Geometry: final body of the model. Coordinates: model frame, mm. A direction names the side the tool comes from. Coordinates: 2 decimals unless noted, no trailing zeros. Order: outer loops, then holes, each group sorted by start corner. A loop starts at its lowest first (then second) coordinate and runs counter-clockwise, first axis right, second up. Notation, with made-up numbers: M 72,59.25 L 115,59.25 A7 cw 115,64.25 Z; hole C 3.25,-8 d4. An arc over 180 degrees is marked long. Use CSV: the item, a comma, the result in double quotes. Start each with the question number.
Q1. Access query for faces 1 (the face through (-4, 3, 5.8)), 2 (the face through (0, 0, 0)). Directions: +Z, -Z, +X, -X, +Y, -Y. A direction counts if a zero-diameter tool reaches every point of the face in a straight line with its end or side. Return the directions, or none.
Q2. Section query B-B, the plane z = 2.75. Output: boundary loops of the cut face in (x, y), and give its area (3 significant figures).
Q3. First-contact query: P1, Ø2, axis at x = -4, y = 1.5, coming from the -Z side; P2, Ø3, axis at x = -2.5, y = 3, coming from the +Z side; P3, Ø2, axis at x = -2.5, y = -0.5, coming from the +Z side; P4, Ø6, axis at x = 2, y = 2.5, coming from the -Z side. Flat tips, straight axial feed; report the tip coordinate or a pass-through.
Q4. Section query A-A, the plane x = 0. Output: boundary loops of the cut face in (y, z) (3 decimals).
Q5. Ray query, probe 1 along Z at (x, y) = (3, -4); probe 2 along X at (y, z) = (3.75, 2.25); probe 3 along Y at (x, z) = (1.75, 4.5). Return the intervals inside material, ascending.
Q6. Section query C-C, the plane z = 1. Output: boundary loops of the cut face in (x, y).
from build123d import *

# Parameters (mm, degrees)
SKETCH7_R           = 0.225
BOSS_EXTRUDE1_DEPTH = 2


with BuildPart() as part:
    # Sketch3 → Revolve1 (revolve)
    with BuildSketch(Plane(origin=(0, 0, 0), x_dir=(0, 0, -1), z_dir=(1, 0, 0)), mode=Mode.PRIVATE) as revolve1_sk:
        Polygon((0, 0), (0, 5.5), (-5.8, 5.2), (-5.8, 0), align=None)
    revolve(revolve1_sk.sketch.rotate(Axis((0, 0, 5.8), (0, 0, -1)), 90), axis=Axis((0, 0, 5.8), (0, 0, -1)))

    # Sketch5 → Revolve2 (revolve)
    with BuildSketch(Plane(origin=(0, 0, 0), x_dir=(0, 0, -1), z_dir=(1, 0, 0)), mode=Mode.PRIVATE) as revolve2_sk:
        Polygon((-5.8, 4.65), (-9.9, 4.5), (-9.9, 0), (-5.8, 0), align=None)
    revolve(revolve2_sk.sketch.rotate(Axis((0, 0, 9.9), (0, 0, -1)), 180), axis=Axis((0, 0, 9.9), (0, 0, -1)))

    # Sketch6 → Revolve3 (revolve)
    with BuildSketch(Plane(origin=(0, 0, 0), x_dir=(0, 0, -1), z_dir=(1, 0, 0))):
        with BuildLine():
            Line((-10.9, 0), (-9.9, 0))
            Line((-9.9, 0), (-9.9, 4.5))
            ThreePointArc((-9.9, 4.5), (-10.646987514, 2.304886114), (-10.9, 0))
        make_face()
    revolve(axis=Axis((0, 0, 0), (0, 0, 1)))

    # Sketch7 → Boss-Extrude1 (add)
    with BuildSketch(Plane(origin=(0, 0, 0), x_dir=(-1, 0, 0), z_dir=(0, 0, -1))):
        with Locations(Location((2.54, 0.048471669, 0), (0, 0, 180))):
            Circle(SKETCH7_R)
        with Locations(Location((0, -2.491528331, 0), (0, 0, 180))):
            Circle(SKETCH7_R)
        with Locations(Location((-2.54, 0.048471669, 0), (0, 0, 180))):
            Circle(SKETCH7_R)
    extrude(amount=BOSS_EXTRUDE1_DEPTH)


solid = part.part
Responses:
1,face 1,"+Z"
1,face 2,"-Z"
2,outline,"C 0,0 d10.72"
2,area,"90.2 mm²"
3,P1,"stops at z = 0"
3,P2,"stops at z = 10.62"
3,P3,"stops at z = 10.79"
3,P4,"stops at z = -2"
4,outline,"M -5.5,0 L -2.717,0 L -2.717,-2 L -2.267,-2 L -2.267,0 L 5.5,0 L 5.2,5.8 L 4.65,5.8 L 4.5,9.9 A10.625 ccw -4.5,9.9 L -4.65,5.8 L -5.2,5.8 Z"
5,probe 1,"z = 0 to 5.8"
5,probe 2,"x = -3.86 to 3.86"
5,probe 3,"y = -4.97 to 4.97"
6,outline,"C 0,0 d10.9"
